The model under review builds one solid part; all positions refer to its coordinate system, in mm. Face numbers are marked on the shaded views. Coordinates: 2 decimals unless noted, no trailing zeros. Loops run counter-clockwise (first coordinate to the right, second up) from the corner with the lowest first, then second, coordinate; pieces in that order, holes last. Notation, with made-up numbers: M -3.5,71.25 L 6.5,71.25 A28 cw 6.5,104.25 Z; hole C -4.75,-14.5 d8. An arc over 180 degrees is marked long. Use one line per item in the form item = value.
```python
from build123d import *

# Parameters (mm, degrees)
F0_R      = 25
F1_DEPTH  = 50
F2_R      = 24.5
F3_DEPTH  = 49
F4_W      = 133.0040432513
F4_H      = 80.2016193047
F5_DEPTH  = 25
F7_DEPTH  = 49
F8_W      = 90.9072607756
F8_H      = 76.9354877993
F9_DEPTH  = 25
F11_R     = 5.0048176475
F11_R_2   = 4.4964097491
F12_DEPTH = 255
F13_DEPTH = 22
F14_R     = 4.5351415883
F15_DEPTH = 500


with BuildPart() as f1:
    # F0 (on Top) → F1 (new body)
    with BuildSketch(Plane.XY):
        Circle(F0_R)
    extrude(amount=F1_DEPTH)

    # F2 (on face) → F3 (cut)
    with BuildSketch(Plane.XY.offset(50)):
        Circle(F2_R)
    extrude(amount=-F3_DEPTH, mode=Mode.SUBTRACT)

    # F4 (on Front) → F5 (cut)
    with BuildSketch(Plane.XZ):
        with Locations((-6.1693545431, 24.7681471519)):
            Rectangle(F4_W, F4_H)
    extrude(amount=-F5_DEPTH, mode=Mode.SUBTRACT)

    # F6 (on face) → F7 (join)
    with BuildSketch(Plane.XY.offset(1)):
        with BuildLine():
            ThreePointArc((-23.7997439297, 0.2099188306), (-23.7849922899, 0.2579040005), (-23.7800096296, 0.307857584))
            ThreePointArc((-23.7800096296, 0.307857584), (-23.7800491855, 0.3123303341), (-23.780167841, 0.3168016851))
            ThreePointArc((-23.780167841, 0.3168016851), (-23.8565770485, 0.4891434991), (-24.0309707308, 0.5607459532))
            ThreePointArc((-24.0309707308, 0.5607459532), (-23.8896091672, 0.4023027599), (-23.7997439297, 0.2099188306))
        make_face()
        with BuildLine():
            ThreePointArc((-23.780167841, 0.3168016851), (-23.7800491855, 0.3123303341), (-23.7800096296, 0.307857584))
            ThreePointArc((-23.7800096296, 0.307857584), (-23.7849922899, 0.2579040005), (-23.7997439297, 0.2099188306))
            ThreePointArc((-23.7997439297, 0.2099188306), (-23.780898653, 0.1315968548), (-23.77078537, 0.0516769082))
            Line((-23.77078537, 0.0516769082), (-23.780167841, 0.3168016851))
        make_face()
        with BuildLine():
            ThreePointArc((-23.77078537, 0.0516769082), (-23.780898653, 0.1315968548), (-23.7997439297, 0.2099188306))
            ThreePointArc((-23.7997439297, 0.2099188306), (-24.1447977278, 0.0810616911), (-24.2525015897, 0.4332919626))
            Line((-24.2525015897, 0.4332919626), (-24.5, 0))
            Line((-24.5, 0), (-23.7689565817, 0))
            Line((-23.7689565817, 0), (-23.77078537, 0.0516769082))
        make_face()
        with BuildLine():
            ThreePointArc((-24.2525015897, 0.4332919626), (-24.1447977278, 0.0810616911), (-23.7997439297, 0.2099188306))
            ThreePointArc((-23.7997439297, 0.2099188306), (-23.8896091672, 0.4023027599), (-24.0309707308, 0.5607459532))
            ThreePointArc((-24.0309707308, 0.5607459532), (-24.1590214746, 0.5270629802), (-24.2525015897, 0.4332919626))
        make_face()
        with BuildLine():
            ThreePointArc((-24.5, 0), (-24.4972731927, -0.3655217092), (-24.489093378, -0.7309620544))
            ThreePointArc((-24.489093378, -0.7309620544), (-23.9792324445, -0.5130551945), (-23.7689565817, 0))
            Line((-23.7689565817, 0), (-24.5, 0))
        make_face()
    extrude(amount=F7_DEPTH)

    # F8 (on Right) → F9 (cut)
    with BuildSketch(Plane.YZ):
        with Locations((-10.7056461275, 28.0342758633)):
            Rectangle(F8_W, F8_H)
    extrude(amount=F9_DEPTH, mode=Mode.SUBTRACT)

    # F10: F1 across face


with BuildPart() as f1_1:
    add(f1.part)
    add(f1.part.mirror(Plane(origin=(0, -18.5631313131, 12.8737373737), x_dir=(0, 1, 0), z_dir=(1, 0, 0))))

    # F11 (on Right) → F12 (join)
    with BuildSketch(Plane.YZ):
        with Locations((0, 25.0316294775)):
            Circle(F11_R)
        with Locations((0, 25.0316294775)):
            Circle(F11_R_2, mode=Mode.SUBTRACT)
    extrude(amount=F12_DEPTH)

    # F11 (on Right) → F13 (cut)
    with BuildSketch(Plane.YZ):
        with Locations((0, 25.0316294775)):
            Circle(F11_R)
        with Locations((0, 25.0316294775)):
            Circle(F11_R_2, mode=Mode.SUBTRACT)
    extrude(amount=F13_DEPTH, mode=Mode.SUBTRACT)

    # F14 (on Right) → F15 (cut)
    with BuildSketch(Plane.YZ):
        with Locations((0, 25.0294525176)):
            Circle(F14_R)
    extrude(amount=F15_DEPTH, mode=Mode.SUBTRACT)


solid = f1_1.part
```
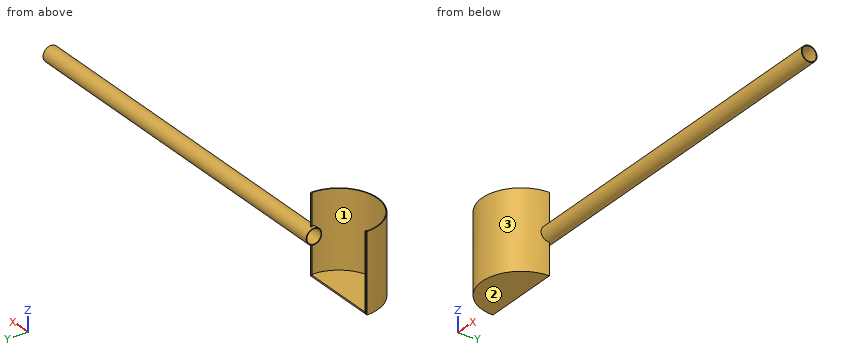
1. Add section A-A (z = 45.5). State the section outline as (x, y) points, then the cut area to 3 significant figures.
Response values:
outline = M -25,0 A25 ccw 25,0 L 24.5,0 L 24.25,0.43 A0.25 ccw 23.78,0.32 L 23.77,0 A0.73 ccw 24.49,-0.73 A24.5 cw -24.49,-0.73 A0.73 ccw -23.77,0 L -23.78,0.32 A0.25 ccw -24.25,0.43 L -24.5,0 Z
area = 40.3 mm^2
2. Insertion check: P1, Ø0.6, axis at x = 24, y = 0.5, coming from the -Z side; P2, Ø12.5, axis at x = 6, y = -7, coming from the +Z side; P3, Ø4, axis at y = -12, z = 36.5, coming from the +X side. Each pin has a flat end and moves straight along its axis. Give the tip position at first contact, or say it passes through.
Response values:
P1 = 1
P2 = 1
P3 = 22.91
3. Add section C-C (x = 0). State the section outline as (y, z) points, then the cut area to 3 significant figures.
Response values:
outline = M -25,0 L 0,0 L 0,1 L -24.5,1 L -24.5,50 L -25,50 Z
area = 49.5 mm^2
4. Add section D-D (x = 45.5). State the section outline as (y, z) points.
Response values:
outline = C 0,25.03 d10.01; hole C 0,25.03 d9.07
5. The part is to be moulded in two halves that separate along X. For the marked faces 1, 2 and 3, say which applies: pulls with the +X half, pulls with the -X half, needs draft (parallel to the pull), parting line crosses it, or undercut.
Response values:
face_1 = undercut
face_2 = needs draft
face_3 = parting line crosses it
6. Wall thickness on line 1 along X through (y, z) = (-1, 15.5); line 2 along Z through (x, y) = (150, 0); line 3 along X through (y, z) = (-6, 35.5): over which ranges is each line inside the solid? List them lowest first. Write a range as from..to.
Response values:
line_1 = -24.98..-24.48, 24.48..24.98
line_2 = 20.03..20.49, 29.56..30.04
line_3 = -24.27..-23.75, 23.75..24.27
7. Add section B-B (y = -12). State the section outline as (x, z) points, then the cut area to 3 significant figures.
Response values:
outline = M -21.93,0 L 21.93,0 L 21.93,50 L 21.36,50 L 21.36,1 L -21.36,1 L -21.36,50 L -21.93,50 Z
area = 99.9 mm^2
